```python
from build123d import *

# Parameters (mm, degrees)
SKETCH_1_W          = 25
SKETCH_1_H          = 20
EXTRUDE_1_DEPTH     = 3
FILLET_1_R          = 5
CUT_EXTRUDE_1_DEPTH = 3
SKETCH_3_W          = 15
SKETCH_3_H          = 3
EXTRUDE_2_DEPTH     = 3
CUT_EXTRUDE_2_DEPTH = 3


with BuildPart() as part:
    # 草图1 → 凸台-拉伸1 (new body)
    with BuildSketch(Plane.XY):
        with BuildLine():
            ThreePointArc((0, 20), (-17.656339801, 9.39434217), (-16.586969757, -11.174633519))
            ThreePointArc((-16.586969757, -11.174633519), (-9.39434217, -17.656339801), (0, -20))
            Line((0, -20), (0, -7.5))
            ThreePointArc((0, -7.5), (-7.5, 0), (0, 7.5))
            Line((0, 7.5), (0, 20))
        make_face()
        with BuildLine():
            ThreePointArc((20, 0), (14.142135624, 14.142135624), (0, 20))
            Line((0, 20), (0, 7.5))
            ThreePointArc((0, 7.5), (5.303300859, 5.303300859), (7.5, 0))
            ThreePointArc((7.5, 0), (5.303300859, -5.303300859), (0, -7.5))
            Line((0, -7.5), (0, -20))
            ThreePointArc((0, -20), (9.39434217, -17.656339801), (16.586969757, -11.174633519))
            ThreePointArc((16.586969757, -11.174633519), (19.127720658, -5.842114551), (20, 0))
        make_face()
        with BuildLine():
            Line((25, 31), (0, 31))
            Line((0, 31), (0, 20))
            ThreePointArc((0, 20), (14.142135624, 14.142135624), (20, 0))
            ThreePointArc((20, 0), (19.127720658, -5.842114551), (16.586969757, -11.174633519))
            Line((16.586969757, -11.174633519), (45, 31))
            Line((45, 31), (25, 31))
        make_face()
        with BuildLine():
            Line((-25, 31), (-45, 31))
            Line((-45, 31), (-16.586969757, -11.174633519))
            ThreePointArc((-16.586969757, -11.174633519), (-17.656339801, 9.39434217), (0, 20))
            Line((0, 20), (0, 31))
            Line((0, 31), (-25, 31))
        make_face()
        with Locations((-12.5, 41)):
            Rectangle(SKETCH_1_W, SKETCH_1_H)
        with Locations((12.5, 41)):
            Rectangle(SKETCH_1_W, SKETCH_1_H)
    extrude(amount=EXTRUDE_1_DEPTH)

    # 圆角1
    fillet_1_edges = [part.edges().sort_by_distance(p)[0] for p in [
        (45, 31, 1.5),
        (-45, 31, 1.5),
    ]]
    fillet(fillet_1_edges, radius=FILLET_1_R)

    # 草图2 → 切除-拉伸1 (cut)
    with BuildSketch(Plane.XY.offset(3)):
        with BuildLine():
            Line((-17.5, 34), (-13.822875656, 34))
            ThreePointArc((-13.822875656, 34), (-12.5, 34.5), (-11.177124344, 34))
            Line((-11.177124344, 34), (-7.5, 34))
            Line((-7.5, 34), (-7.5, 31))
            Line((-7.5, 31), (-11.177124344, 31))
            ThreePointArc((-11.177124344, 31), (-12.5, 30.5), (-13.822875656, 31))
            Line((-13.822875656, 31), (-17.5, 31))
            Line((-17.5, 31), (-17.5, 34))
        make_face()
        with BuildLine():
            Line((7.5, 34), (11.177124344, 34))
            ThreePointArc((11.177124344, 34), (12.5, 34.5), (13.822875656, 34))
            Line((13.822875656, 34), (17.5, 34))
            Line((17.5, 34), (17.5, 31))
            Line((17.5, 31), (13.822875656, 31))
            ThreePointArc((13.822875656, 31), (12.5, 30.5), (11.177124344, 31))
            Line((11.177124344, 31), (7.5, 31))
            Line((7.5, 31), (7.5, 34))
        make_face()
    extrude(amount=-CUT_EXTRUDE_1_DEPTH, mode=Mode.SUBTRACT)

    # 草图3 → 凸台-拉伸2 (add)
    with BuildSketch(Plane.XY.offset(3)):
        with Locations((-13.5, 52.5)):
            Rectangle(SKETCH_3_W, SKETCH_3_H)
        with Locations((13.5, 52.5)):
            Rectangle(SKETCH_3_W, SKETCH_3_H)
    extrude(amount=-EXTRUDE_2_DEPTH)

    # 草图4 → 切除-拉伸2 (cut)
    with BuildSketch(Plane.XY.offset(3)):
        Polygon((-15.75, 54), (-15.75, 48), (-17.75, 48), (-17.75, 43), (-15.75, 43), (-15.75, 41), (-11.25, 41), (-11.25, 43), (-9.25, 43), (-9.25, 48), (-11.25, 48), (-11.25, 54), align=None)
        Polygon((11.25, 48), (11.25, 54), (15.75, 54), (15.75, 48), (17.75, 48), (17.75, 43), (15.75, 43), (15.75, 41), (11.25, 41), (11.25, 43), (9.25, 43), (9.25, 48), align=None)
    extrude(amount=-CUT_EXTRUDE_2_DEPTH, mode=Mode.SUBTRACT)


solid = part.part
```
Source: CAD feature listing. Evaluate the final solid. Frame: model axes, mm. A direction names the side the tool comes from. Coordinates: 2 decimals unless noted, no trailing zeros. Write each loop counter-clockwise with the first axis right and the second up, starting at its lowest first coordinate (ties: lowest second). Pieces come first, ordered by that corner, then holes. Notation, with made-up numbers: (-18, -38) -> (7, -38) arc R29 ccw to (7, -8) -> close; hole circle Ø1 at (69.5, 50.5). An arc over 180 degrees is marked (long way). Return JSON: item names as keys, results as strings. Group by question number.
1) Section query B-B, the plane z = 1.1. State how many separate pieces and enclosed holes the cut face has, plus the area to 3 significant figures.
2) Section query D-D, the plane y = 28.5. Return loops of the section in (x, z).
3) Section query A-A, the plane y = 46. Return loops of the section in (x, z).
4) Ray query, line 1 along X through (y, z) = (32, 2.6); line 2 along Y through (x, z) = (-16, 0.75); line 3 along Y through (x, z) = (11, 1.2). Return the intervals inside material, ascending.
5) Contact query for flat-ended pins moving along their axis: P1, Ø1.5, axis at y = 52, z = 2, coming from the -X side; P2, Ø0.6, axis at y = 41.5, z = 2, coming from the -X side; P3, Ø0.9, axis at y = 52, z = 2, coming from the +X side. Output: stop coordinate, or through.
6) Mould query, pull axis Y, two halves, no side actions, for faces 1 (the face through (9.25, 45, 2)), 2 (the face through (21, 52, 2)), 3 (the face through (0, 51, 1)). Classes: +Y half, -Y half, draft (parallel to the pull), parting line (faces both ways), or undercut.
7) Set-up query: faces 4 (the face through (25, 41, 1)), 5 (the face through (14, 41, 2)), 6 (the face through (-10, 48, 2)). Return all of +Z, -Z, +X, -X, +Y, -Y with unobstructed straight access to the full face (end or side cutting, diameter ignored); none if empty.
8) Section query C-C, the plane x = -34. Return loops of the section in (y, z), plus the area to 3 significant figures.
From the geometry:
{
 "1": {"separate pieces": "1", "enclosed holes": "3", "area": "3,460 mm²"},
 "2": {"outline": "(-39.93, 0) -> (39.93, 0) -> (39.93, 3) -> (-39.93, 3) -> close"},
 "3": {"outline": "(-25, 0) -> (-17.75, 0) -> (-17.75, 3) -> (-25, 3) -> close; (-9.25, 0) -> (9.25, 0) -> (9.25, 3) -> (-9.25, 3) -> close; (17.75, 0) -> (25, 0) -> (25, 3) -> (17.75, 3) -> close"},
 "4": {"line 1": "-25 to -17.5, -7.5 to 7.5, 17.5 to 25", "line 2": "-12 to 31, 34 to 43, 48 to 54", "line 3": "-16.7 to 31, 34 to 43, 48 to 54"},
 "5": {"P1": "x = -21", "P2": "x = -25", "P3": "x = 21"},
 "6": {"face 1": "undercut", "face 2": "draft", "face 3": "+Y half"},
 "7": {"face 4": "+Z, -Z, +X, +Y", "face 5": "+Z, -Z, +Y", "face 6": "+Z, -Z"},
 "8": {"outline": "(14.67, 0) -> (31, 0) -> (31, 3) -> (14.67, 3) -> close", "area": "49.0 mm²"}
}
